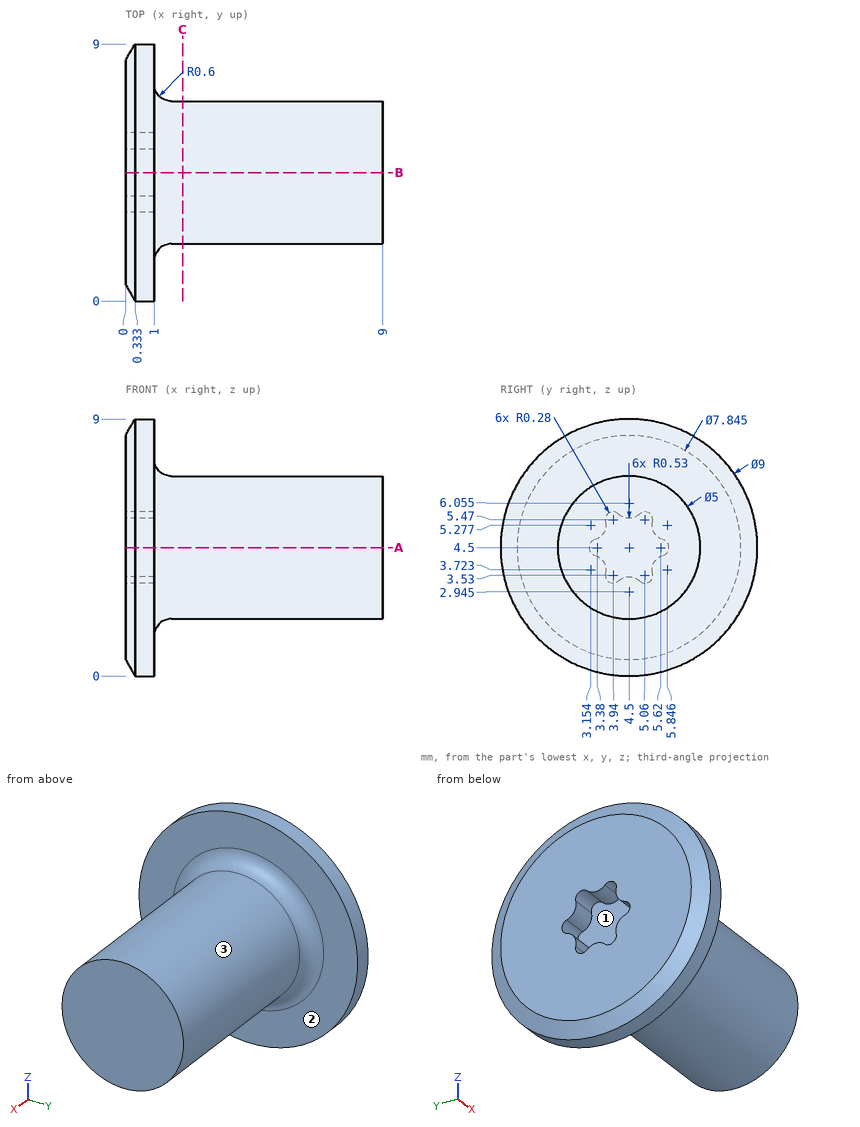
Geometry: see drawing. Coordinates: mm, zero at the bounding-box minimum. Coordinates: 2 decimals unless noted, no trailing zeros. Order: outer loops, then holes, each group sorted by start corner. A loop starts at its lowest first (then second) coordinate and runs counter-clockwise, first axis right, second up. Notation, with made-up numbers: (9.25, -1) - (46.25, -1) arc R29 ccw to (46.25, 23) - close; hole circle Ø1 at (-34.75, 75). An arc over 180 degrees is marked (long way). Return JSON: item names as keys, results as strings.
Q1. Cut plane C-C (x = 2). Return loops of the section in (y, z).
The answers:
{"outline": "circle Ø5 at (4.5, 4.5)"}
Q2. First-contact query: pin 1 (1 mm diameter, centred on x = 7, z = 7, fed in from -Y); pin 2 (4 mm diameter, centred on x = 7.5, z = 8, fed in from +Y); pin 3 (3 mm diameter, centred on x = 5, z = 2, fed in from +Y). Flat tips, straight axial feed; report the tip coordinate or a pass-through.
The answers:
{"pin 1": "stops at y = 3", "pin 2": "stops at y = 6.5", "pin 3": "stops at y = 6.79"}
Q3. Cut plane B-B (y = 4.5). Return loops of the section in (x, z) (1 decimal), then the cut area to 3 significant figures.
The answers:
{"outline": "(0, 0.6) - (0.3, 0) - (1, 0) - (1, 1.4) arc R0.6 cw to (1.6, 2) - (9, 2) - (9, 7) - (1.6, 7) arc R0.6 cw to (1, 7.6) - (1, 9) - (0.3, 9) - (0, 8.4) - (0, 5.5) - (1, 5.5) - (1, 3.5) - (0, 3.5) - close", "area": "46.9 mm2"}
Q4. Draft query along Y for the marked faces 1, 2 and 3. Return one class per face: +Y half, -Y half, draft (parallel to the pull), parting line (faces both ways), or undercut.
The answers:
{"face 1": "undercut", "face 2": "draft", "face 3": "parting line"}
Q5. Ray query, probe 1 along Y at (x, z) = (3, 4.5); probe 2 along X at (y, z) = (4.5, 4). Return the intervals inside material, ascending.
The answers:
{"probe 1": "y = 2 to 7", "probe 2": "x = 1 to 9"}
Q6. Cut plane A-A (z = 4.5). Return loops of the section in (x, y).
The answers:
{"outline": "(0, 0.58) - (0.33, 0) - (1, 0) - (1, 1.4) arc R0.6 cw to (1.6, 2) - (9, 2) - (9, 7) - (1.6, 7) arc R0.6 cw to (1, 7.6) - (1, 9) - (0.33, 9) - (0, 8.42) - (0, 5.9) - (1, 5.9) - (1, 3.1) - (0, 3.1) - close"}
